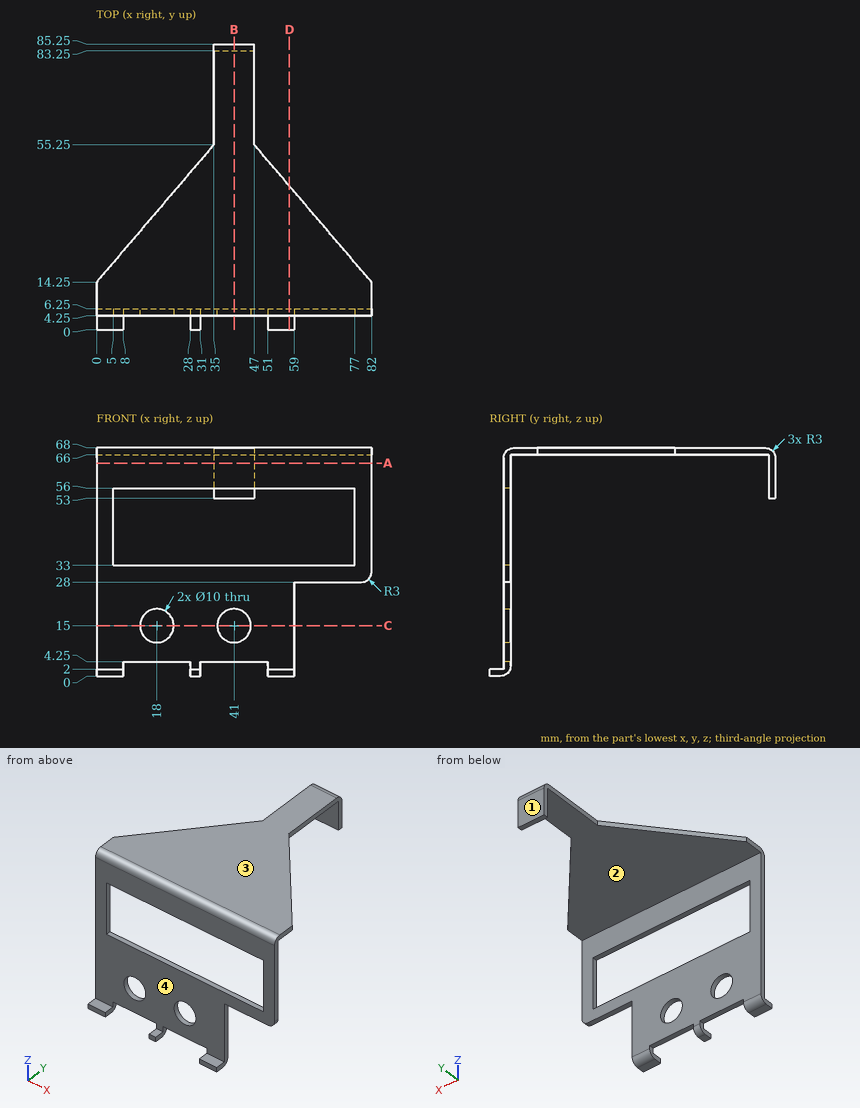
Design review of the part shown in the three views and the two pictorial views. Dimensions are in mm from the part's minimum x, y and z. Coordinates: 2 decimals unless noted, no trailing zeros. Order: outer loops, then holes, each group sorted by start corner. A loop starts at its lowest first (then second) coordinate and runs counter-clockwise, first axis right, second up.
1) Take a section at C-C, the plane z = 15. Give the boundary of the cut face in (x, y).
2) Take a section at D-D, the plane x = 57.5. Give the boundary of the cut face in (y, z).
3) Mouldability with a two-part tool opening along Y and no side actions: class the marked faces 1, 2, 3 and 4 as +Y half, -Y half, draft (parallel to the pull), parting line (faces both ways), or undercut.
4) Take a section at B-B, the plane x = 41. Give the boundary of the cut face in (y, z), and give its area (3 significant figures).
5) Take a section at A-A, the plane z = 63.5. Give the boundary of the cut face in (x, y), and give its area (3 significant figures).
6) Clearance check with flat-ended pins moving along their axes: pin 1 (6 mm diameter, centred on x = 41, y = 20, fed in from -Z); pin 2 (1.6 mm diameter, centred on x = 45, y = 5, fed in from -Z); pin 3 (11.5 mm diameter, centred on x = 18, z = 15, fed in from +Y); pin 4 (2 mm diameter, centred on y = 2, z = 2, fed in from -X). State where each tip first meets the part, or that it passes through.
7) Wall thickness on line 1 along Z through (x, y) = (41, 4.95); line 2 along Z through (x, y) = (18, 5.3); line 3 along Y through (x, z) = (38, 20.5): over which ranges is each line inside the solid? List them lowest first.
Returned:
1. outline: (0, 4.25) - (13, 4.25) - (13, 6.25) - (0, 6.25) - close; (23, 4.25) - (36, 4.25) - (36, 6.25) - (23, 6.25) - close; (46, 4.25) - (59, 4.25) - (59, 6.25) - (46, 6.25) - close
2. outline: (0, 0) - (3.25, 0) arc R3 ccw to (6.25, 3) - (6.25, 33) - (4.25, 33) - (4.25, 2) - (0, 2) - close; (4.25, 56) - (6.25, 56) - (6.25, 66) - (42.95, 66) - (42.95, 68) - (7.25, 68) arc R3 ccw to (4.25, 65) - close
3. face 1: +Y half
3. face 2: undercut
3. face 3: draft
3. face 4: -Y half
4. outline: (4.25, 4.25) - (6.25, 4.25) - (6.25, 10) - (4.25, 10) - close; (4.25, 20) - (6.25, 20) - (6.25, 33) - (4.25, 33) - close; (4.25, 56) - (6.25, 56) - (6.25, 66) - (83.25, 66) - (83.25, 53) - (85.25, 53) - (85.25, 65) arc R3 ccw to (82.25, 68) - (7.25, 68) arc R3 ccw to (4.25, 65) - close
4. area: 242 mm2
5. outline: (0, 4.25) - (82, 4.25) - (82, 6.25) - (0, 6.25) - close; (35, 83.25) - (47, 83.25) - (47, 85.25) - (35, 85.25) - close
5. area: 188 mm2
6. pin 1: stops at z = 66
6. pin 2: stops at z = 4.25
6. pin 3: stops at y = 6.25
6. pin 4: stops at x = 0
7. line 1: z = 4.25 to 10, 20 to 33, 56 to 66.93
7. line 2: z = 4.25 to 10, 20 to 33, 56 to 67.28
7. line 3: y = 4.25 to 6.25
